```python
from build123d import *

# Parameters (mm, degrees)
SALIENTE_EXTRUIR1_DEPTH = 3


with BuildPart() as part:
    # Model → Saliente-Extruir1 (new body)
    with BuildSketch(Plane.XY):
        with BuildLine():
            Line((47.379734173, 293.880494369), (50.419280292, 293.880494369))
            ThreePointArc((50.419280292, 293.880494369), (51.126387073, 293.58760115), (51.419280292, 292.880494369))
            Line((51.419280292, 292.880494369), (51.419280292, 282.514242123))
            Line((51.419280292, 282.514242123), (53.269280292, 282.514242123))
            ThreePointArc((53.269280292, 282.514242123), (53.363243785, 282.877719909), (53.621589895, 283.150121316))
            ThreePointArc((53.621589895, 283.150121316), (53.770849393, 283.175830273), (53.895329391, 283.089551201))
            Line((53.895329391, 283.089551201), (54.919280292, 281.514242123))
            Line((54.919280292, 281.514242123), (54.919280292, 279.062526812))
            ThreePointArc((54.919280292, 279.062526812), (54.040600635, 276.941206469), (51.919280292, 276.062526812))
            Line((51.919280292, 276.062526812), (46.919280292, 276.062526812))
            ThreePointArc((46.919280292, 276.062526812), (46.212173511, 276.355420031), (45.919280292, 277.062526812))
            Line((45.919280292, 277.062526812), (45.919280292, 287.014242123))
            Line((45.919280292, 287.014242123), (42.919280292, 287.014242123))
            Line((42.919280292, 287.014242123), (42.919280292, 282.514242123))
            Line((42.919280292, 282.514242123), (36.919280292, 282.514242123))
            Line((36.919280292, 282.514242123), (36.919280292, 287.014242123))
            Line((36.919280292, 287.014242123), (33.919280292, 287.014242123))
            Line((33.919280292, 287.014242123), (33.919280292, 282.514242123))
            Line((33.919280292, 282.514242123), (20.919280292, 282.514242123))
            Line((20.919280292, 282.514242123), (20.919280292, 287.014242123))
            Line((20.919280292, 287.014242123), (17.919280292, 287.014242123))
            Line((17.919280292, 287.014242123), (17.919280292, 277.062526812))
            ThreePointArc((17.919280292, 277.062526812), (17.58071812, 276.312526812), (16.794280292, 276.070370071))
            ThreePointArc((16.794280292, 276.070370071), (8.920876277, 284.83029571), (16.458826411, 293.880494369))
            ThreePointArc((16.458826411, 293.880494369), (16.927302549, 293.845714495), (17.328205845, 293.600855192))
            Line((17.328205845, 293.600855192), (17.626387073, 293.302673965))
            ThreePointArc((17.626387073, 293.302673965), (17.843159824, 292.978250616), (17.919280292, 292.595567183))
            Line((17.919280292, 292.595567183), (20.519280292, 292.595567183))
            ThreePointArc((20.519280292, 292.595567183), (20.802123004, 292.478409896), (20.919280292, 292.195567183))
            Line((20.919280292, 292.195567183), (20.919280292, 291.995567183))
            ThreePointArc((20.919280292, 291.995567183), (21.036437579, 291.712724471), (21.319280292, 291.595567183))
            Line((21.319280292, 291.595567183), (42.119280292, 291.595567183))
            ThreePointArc((42.119280292, 291.595567183), (42.402123004, 291.712724471), (42.519280292, 291.995567183))
            Line((42.519280292, 291.995567183), (42.519280292, 292.195567183))
            ThreePointArc((42.519280292, 292.195567183), (42.636437579, 292.478409896), (42.919280292, 292.595567183))
            Line((42.919280292, 292.595567183), (45.919280292, 292.595567183))
            ThreePointArc((45.919280292, 292.595567183), (45.995400759, 292.978250616), (46.212173511, 293.302673965))
            Line((46.212173511, 293.302673965), (46.510354738, 293.600855192))
            ThreePointArc((46.510354738, 293.600855192), (46.911258035, 293.845714495), (47.379734173, 293.880494369))
        make_face()
    extrude(amount=SALIENTE_EXTRUIR1_DEPTH)


solid = part.part
```
The listing builds one solid part. Answer for the finished solid, in the listing's coordinates (mm). A direction names the side the tool comes from. Give positions to 0.01 mm unless a question says otherwise; leave off trailing zeros. Order: outer loops, then holes, each group sorted by start corner. A loop starts at its lowest first (then second) coordinate and runs counter-clockwise, first axis right, second up. Notation, with made-up numbers: (63, 25.5) - (85, 25.5) arc R23 cw to (85, 42.5) - close; hole circle Ø8 at (16, -7.75). An arc over 180 degrees is marked (long way). Answer in a Markdown table with one row per item. Add a question column.
Q1. The part is cut by section A-A (y = 284). Determine the outline of the cut face in (x, z), then the cut area to 3 significant figures.
Q2. Find the intervals of material crossed by line 1 along X through (y, z) = (286, 0.3); line 2 along Y through (x, z) = (24.5, 0.8); line 3 along X through (y, z) = (278.5, 0.3), in increasing order. Write a range as [from, to].
Q3. Which of the six approach directions +Z, -Z, +X, -X, +Y, -Y give full straight-line access (tool end or side, diameter ignored) to faces 4 (the flat face through (45.919, 282, 1)), 5 (the flat face through (19, 292.596, 1))?
Q4. The part is cut by section B-B (y = 280.5). Determine the outline of the cut face in (x, z).
Q5. The part is cut by section C-C (x = 29). Determine the outline of the cut face in (y, z).
Q6. For a pull along X with two mould halves and no side action, classify faces 1 (the flat face through (17.919, 282, 1)), 2 (the flat face through (54.4, 282.31, 1.48)), 3 (the cylindrical face through (8.926, 284.651, 1.479)) as released by +X, released by -X, zero draft, split by the parting line, or undercut.
Q7. Given P1, Ø0.9, axis at x = 38.5, z = 1, coming from the -Y side; P2, Ø1.5, axis at y = 285, z = 2, coming from the +X side; P3, Ø1.5, axis at x = 41, z = 0.5, coming from the +Y side; P4, Ø3, axis at x = 41, y = 284.5, coming from the -Z side, each flat-ended and moving along its own axis, determine where each tip first touches the part or whether it passes through.
Q8. The part is cut by section D-D (y = 278.25). Determine the outline of the cut face in (x, z).
Determined:
| question | item | result |
|---|---|---|
| 1 | outline | (8.97, 0) - (17.92, 0) - (17.92, 3) - (8.97, 3) - close; (20.92, 0) - (33.92, 0) - (33.92, 3) - (20.92, 3) - close; (36.92, 0) - (42.92, 0) - (42.92, 3) - (36.92, 3) - close; (45.92, 0) - (51.42, 0) - (51.42, 3) - (45.92, 3) - close |
| 1 | area | 100 mm² |
| 2 | line 1 | x = [8.98, 17.92], [20.92, 33.92], [36.92, 42.92], [45.92, 51.42] |
| 2 | line 2 | y = [282.51, 291.6] |
| 2 | line 3 | x = [11.69, 17.92], [45.92, 54.87] |
| 3 | face 4 | +Z, -Z, -Y |
| 3 | face 5 | +Z, -Z, +Y |
| 4 | outline | (10.12, 0) - (17.92, 0) - (17.92, 3) - (10.12, 3) - close; (45.92, 0) - (54.92, 0) - (54.92, 3) - (45.92, 3) - close |
| 5 | outline | (282.51, 0) - (291.6, 0) - (291.6, 3) - (282.51, 3) - close |
| 6 | face 1 | undercut |
| 6 | face 2 | released by +X |
| 6 | face 3 | released by -X |
| 7 | P1 | stops at y = 282.51 |
| 7 | P2 | stops at x = 51.42 |
| 7 | P3 | stops at y = 291.6 |
| 7 | P4 | stops at z = 0 |
| 8 | outline | (11.97, 0) - (17.92, 0) - (17.92, 3) - (11.97, 3) - close; (45.92, 0) - (54.81, 0) - (54.81, 3) - (45.92, 3) - close |
